```python
from build123d import *

# Parameters (mm, degrees)
SKETCH1_R           = 4.05
BOSS_EXTRUDE1_DEPTH = 20
FILLET1_R           = 1
CHAMFER2_SIZE       = 2
SKETCH7_R           = 2.65
CUT_EXTRUDE8_DEPTH  = 40
SKETCH8_R           = 2.65
CUT_EXTRUDE9_DEPTH  = 40
SKETCH9_R           = 5.5
CUT_EXTRUDE10_DEPTH = 40
SKETCH10_R          = 5.5
CUT_EXTRUDE11_DEPTH = 40


with BuildPart() as part:
    # Sketch1 → Boss-Extrude1 (new body)
    with BuildSketch(Plane(origin=(0, 0, 0), x_dir=(1, 0, 0), z_dir=(0, 1, 0))):
        with BuildLine():
            Line((-20, 40), (20, 40))
            Line((20, 40), (20, -10))
            ThreePointArc((20, -10), (17.071067812, -17.071067812), (10, -20))
            Line((10, -20), (-40, -20))
            Line((-40, -20), (-40, 20))
            Line((-40, 20), (-20, 20))
            Line((-20, 20), (-20, 40))
        make_face()
        with Locations(Location((0, 0, 0), (0, 0, 270))):
            Circle(SKETCH1_R, mode=Mode.SUBTRACT)
    extrude(amount=BOSS_EXTRUDE1_DEPTH)

    # Fillet1
    fillet1_edges = [part.edges().sort_by_distance(p)[0] for p in [
        (0, 20, -4.05),
    ]]
    fillet(fillet1_edges, radius=FILLET1_R)

    # Chamfer2
    chamfer2_edges = [part.edges().sort_by_distance(p)[0] for p in [
        (-15, 20, 20),
        (17.071067812, 20, 17.071067812),
        (20, 20, -15),
        (20, 0, -15),
        (17.071067812, 0, 17.071067812),
        (-15, 0, 20),
    ]]
    chamfer(chamfer2_edges, length=CHAMFER2_SIZE)

    # Sketch7 → Cut-Extrude8 (cut)
    with BuildSketch(Plane.ZY.offset(20)):
        with Locations((-30, 10)):
            Circle(SKETCH7_R)
    extrude(amount=-CUT_EXTRUDE8_DEPTH, mode=Mode.SUBTRACT)

    # Sketch8 → Cut-Extrude9 (cut)
    with BuildSketch(Plane(origin=(0, 0, -20), x_dir=(-1, 0, 0), z_dir=(0, 0, -1))):
        with Locations((30, 10)):
            Circle(SKETCH8_R)
    extrude(amount=-CUT_EXTRUDE9_DEPTH, mode=Mode.SUBTRACT)

    # Sketch9 → Cut-Extrude10 (cut)
    with BuildSketch(Plane.ZY.offset(9)):
        with Locations((-30, 10)):
            Circle(SKETCH9_R)
    extrude(amount=-CUT_EXTRUDE10_DEPTH, mode=Mode.SUBTRACT)

    # Sketch10 → Cut-Extrude11 (cut)
    with BuildSketch(Plane(origin=(0, 0, -9), x_dir=(-1, 0, 0), z_dir=(0, 0, -1))):
        with Locations((30, 10)):
            Circle(SKETCH10_R)
    extrude(amount=-CUT_EXTRUDE11_DEPTH, mode=Mode.SUBTRACT)


solid = part.part
```
For this review, take the finished solid that the model builds, in its own axes (mm). A direction names the side the tool comes from. Coordinates: 2 decimals unless noted, no trailing zeros. Write each loop counter-clockwise with the first axis right and the second up, starting at its lowest first coordinate (ties: lowest second). Pieces come first, ordered by that corner, then holes. Notation, with made-up numbers: (54, 81) - (98, 81) arc R9 cw to (98, 96) - close; hole circle Ø1 at (71, -36.5). An arc over 180 degrees is marked (long way). Put each result on its own line as item: value.
1. Machinability: for faces 1 (the flat face through (-20, 8, -28)), 2 (the cylindrical face through (5.297, 10.242, -35.495)), 3 (the flat face through (-31, 13, -9)), which of the approach directions +Z, -Z, +X, -X, +Y, -Y give a long, thin tool a straight path to every point of the face, cutting with its end or side? Answer none if there is none.
Values found:
face 1: -Z, -X, +Y, -Y
face 2: +X
face 3: +Z
2. Wall thickness on probe 1 along Y at (x, z) = (-30, 2); probe 2 along Y at (x, z) = (-30, -16.75); probe 3 along Z at (x, y) = (-30.5, 6.5): over which ranges is each line inside the solid? List them lowest first.
Values found:
probe 1: 0 to 4.5, 15.5 to 20
probe 2: 0 to 7.35, 12.65 to 20
probe 3: -20 to -9
3. Mouldability with a two-part tool opening along Y and no side actions: class faces 4 (the flat face through (0, 10, -40)), 5 (the cylindrical face through (-14.577, 10.117, -32.647)), 6 (the flat face through (-15, 1, 19)) as released by +Y, released by -Y, zero draft, split by the parting line, or undercut.
Values found:
face 4: zero draft
face 5: undercut
face 6: released by -Y
4. Add section D-D, the plane z = -30. Give the boundary of the cut face in (x, y), then the cut area to 3 significant figures.
Values found:
outline: (-20, 0) - (18, 0) - (20, 2) - (20, 4.5) - (-9, 4.5) - (-9, 7.35) - (-20, 7.35) - close; (-20, 12.65) - (-9, 12.65) - (-9, 15.5) - (20, 15.5) - (20, 18) - (18, 20) - (-20, 20) - close
area: 419 mm²
5. For pin 1 (12 mm diameter, centred on x = -28, y = 10, fed in from +Z); pin 2 (9 mm diameter, centred on x = -30, y = 10, fed in from -Z); pin 3 (3.5 mm diameter, centred on y = 8, z = -32, fed in from +X); pin 4 (7 mm diameter, centred on x = -30, y = 10, fed in from +Z), all flat-tipped, find the tip position at first contact; note any pin that passes through.
Values found:
pin 1: z = 20
pin 2: z = -20
pin 3: x = -9
pin 4: z = -9
6. Add section C-C, the plane y = 10. Give the boundary of the cut face in (x, z), then the cut area to 3 significant figures.
Values found:
outline: (-40, -20) - (-32.65, -20) - (-32.65, -9) - (-35.5, -9) - (-35.5, 20) - (-40, 20) - close; (-27.35, -20) - (-20, -20) - (-20, -27.35) - (-9, -27.35) - (-9, -24.5) - (20, -24.5) - (20, 10) arc R10 ccw to (10, 20) - (-24.5, 20) - (-24.5, -9) - (-27.35, -9) - close; (-20, -40) - (20, -40) - (20, -35.5) - (-9, -35.5) - (-9, -32.65) - (-20, -32.65) - close; hole circle Ø8.1 at (0, 0)
area: 2,370 mm²
7. Add section A-A, the plane z = 0. Give the boundary of the cut face in (x, y).
Values found:
outline: (-40, 0) - (-4.05, 0) - (-4.05, 19) arc R1 ccw to (-5.05, 20) - (-40, 20) - close; (4.05, 0) - (18, 0) - (20, 2) - (20, 18) - (18, 20) - (5.05, 20) arc R1 ccw to (4.05, 19) - close; hole circle Ø11 at (-30, 10)
8. Add section B-B, the plane x = 0. Give the boundary of the cut face in (y, z).
Values found:
outline: (0, -40) - (20, -40) - (20, -5.05) arc R1 ccw to (19, -4.05) - (0, -4.05) - close; (0, 4.05) - (19, 4.05) arc R1 ccw to (20, 5.05) - (20, 18) - (18, 20) - (2, 20) - (0, 18) - close; hole circle Ø11 at (10, -30)
